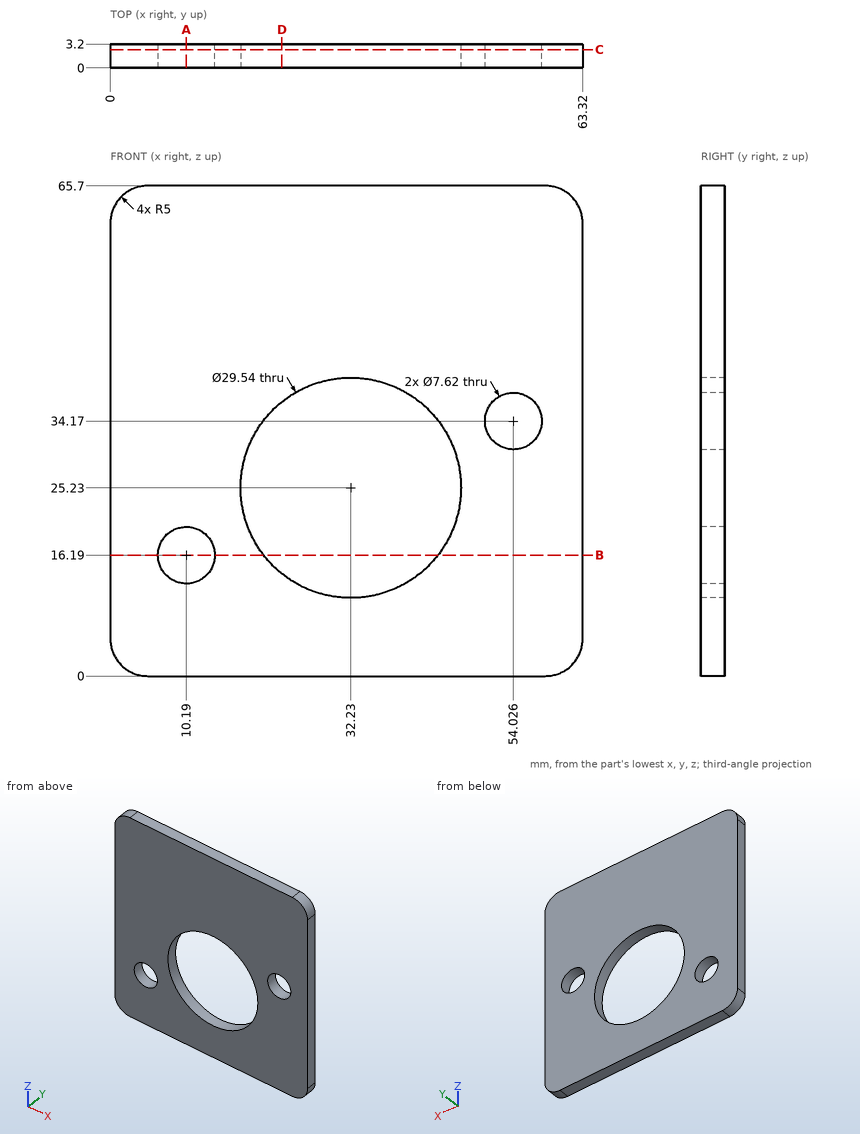
Study the drawing (mm; zero at the part's minimum x, y, z) and answer. Coordinates: 2 decimals unless noted, no trailing zeros. Write each loop counter-clockwise with the first axis right and the second up, starting at its lowest first coordinate (ties: lowest second). Pieces come first, ordered by that corner, then holes. Notation, with made-up numbers: M 31,71.5 L 49,71.5 A22 ccw 49,106.5 Z; hole C 47,-9.75 d3. An arc over 180 degrees is marked long. Write each question's results on one line, items separated by ' | '.
Item 1: The part is cut by section A-A on x = 10.19. Determine the outline of the cut face in (y, z), and give its area (3 significant figures).
Answer below:
outline: M 0,0 L 3.2,0 L 3.2,12.38 L 0,12.38 Z; M 0,20 L 3.2,20 L 3.2,65.7 L 0,65.7 Z | area: 186 mm2
Item 2: The part is cut by section B-B on z = 16.19. Determine the outline of the cut face in (x, y).
Answer below:
outline: M 0,0 L 6.38,0 L 6.38,3.2 L 0,3.2 Z; M 14,0 L 20.55,0 L 20.55,3.2 L 14,3.2 Z; M 43.91,0 L 63.32,0 L 63.32,3.2 L 43.91,3.2 Z
Item 3: The part is cut by section C-C on y = 2.45. Determine the outline of the cut face in (x, z), and give its area (3 significant figures).
Answer below:
outline: M 0,5 A5 ccw 5,0 L 58.32,0 A5 ccw 63.32,5 L 63.32,60.7 A5 ccw 58.32,65.7 L 5,65.7 A5 ccw 0,60.7 Z; hole C 10.19,16.19 d7.62; hole C 32.23,25.23 d29.54; hole C 54.03,34.17 d7.62 | area: 3,360 mm2
Item 4: The part is cut by section D-D on x = 23. Determine the outline of the cut face in (y, z).
Answer below:
outline: M 0,0 L 3.2,0 L 3.2,13.7 L 0,13.7 Z; M 0,36.76 L 3.2,36.76 L 3.2,65.7 L 0,65.7 Z
Item 5: Given P1, Ø1.5, axis at x = 8.5, y = 2.5, coming from the -Z side, flat-ended and moving along its own axis, determine where the tip first touches the part or whether it passes through.
Answer below:
P1: z = 0
Item 6: Consider probe 1 along Z at (x, y) = (10.19, 1.35); probe 2 along X at (y, z) = (2.45, 19); probe 3 along X at (y, z) = (1.55, 34) (1 decimal). Determine where each line is inside the solid, lowest interval first. Write a range as [from, to].
Answer below:
probe 1: [0, 12.38], [20, 65.7] | probe 2: [0, 7.62], [12.76, 18.84], [45.62, 63.32] | probe 3: [0, 20.3], [44.1, 50.2], [57.8, 63.3]
